Can you work these out from the model? Positions are in its coordinate system, mm. A direction names the side the tool comes from. Coordinates: 2 decimals unless noted, no trailing zeros. Loops run counter-clockwise (first coordinate to the right, second up) from the corner with the lowest first, then second, coordinate; pieces in that order, holes last.
```python
from build123d import *

# Parameters (mm, degrees)
BOX010_W          = 30
BOX010_H          = 9
BOX010_DEPTH      = 15
BOX011_W          = 31.5
BOX011_H          = 16
BOX011_DEPTH      = 12
CYLINDER_R        = 1.75
CYLINDER_DEPTH    = 10
CYLINDER001_R     = 1.75
CYLINDER001_DEPTH = 10
BOX009_W          = 44
BOX009_H          = 3
BOX009_DEPTH      = 17


with BuildPart() as cube010:
    # Box010 → Box010 (new body)
    with BuildSketch(Plane(origin=(43, -107, 23), x_dir=(1, 0, 0), z_dir=(0, 0, 1))):
        with Locations((15, 4.5)):
            Rectangle(BOX010_W, BOX010_H)
    extrude(amount=BOX010_DEPTH)


with BuildPart() as cube011:
    # Box011 → Box011 (new body)
    with BuildSketch(Plane(origin=(42, -95, 22), x_dir=(1, 0, 0), z_dir=(0, 0, 1))):
        with Locations((15.75, 8)):
            Rectangle(BOX011_W, BOX011_H)
    extrude(amount=BOX011_DEPTH)


with BuildPart() as cylinder:
    # Cylinder → Cylinder (new body)
    with BuildSketch(Plane(origin=(40, -91, 26.5), x_dir=(1, 0, 0), z_dir=(0, -1, 0))):
        Circle(CYLINDER_R)
    extrude(amount=CYLINDER_DEPTH)


with BuildPart() as fusion003:
    # Cylinder001 → Cylinder001 (new body)
    with BuildSketch(Plane(origin=(76.5, -91, 26.5), x_dir=(1, 0, 0), z_dir=(0, -1, 0))):
        Circle(CYLINDER001_R)
    extrude(amount=CYLINDER001_DEPTH)

    # Fusion003: union Cylinder
    add(cylinder.part)


with BuildPart() as fusion003_1:
    # Fusion003 placement: moved
    add(fusion003.part.moved(Location((-0.5, 0, 0))))


with BuildPart() as f_4p:
    # Box009 → Box009 (new body)
    with BuildSketch(Plane(origin=(36, -98, 19), x_dir=(1, 0, 0), z_dir=(0, 0, 1))):
        with Locations((22, 1.5)):
            Rectangle(BOX009_W, BOX009_H)
    extrude(amount=BOX009_DEPTH)

    # Fusion004: union Cube010, Cube011, Fusion003
    add(cube010.part)
    add(cube011.part)
    add(fusion003_1.part)


with BuildPart() as f_4p_1:
    # Fusion004 placement: moved
    add(f_4p.part.moved(Location((-5, 0, 0))))


solid = f_4p_1.part
```
Item 1: Suppose I cut it at C-C, the plane x = 34.5. Please give me the cut outline in (y, z), plus the area to 3 significant figures.
Results are:
outline: (-101, 24.75) - (-98, 24.75) - (-98, 19) - (-95, 19) - (-95, 24.75) - (-91, 24.75) - (-91, 28.25) - (-95, 28.25) - (-95, 36) - (-98, 36) - (-98, 28.25) - (-101, 28.25) - close
area: 75.5 mm2
Item 2: Suppose I cut it at B-B, the plane y = -100.5. Please give me the cut outline in (x, z), plus the area to 3 significant figures.
Results are:
outline: circle Ø3.5 at (34.5, 26.5); (38, 23) - (68, 23) - (68, 38) - (38, 38) - close; circle Ø3.5 at (71, 26.5)
area: 469 mm2
Item 3: I need wall thicknesses on line 1 along Z through (x, y) = (59.5, -99); line 2 along Z through (x, y) = (68, -88.5); line 3 along X through (y, z) = (-91, 24.5). Which ranges of each line are inside material? Lowest first, please.
Results are:
line 1: z = 23 to 38
line 2: z = 22 to 34
line 3: x = 37 to 68.5
Item 4: I'm going to push flat-ended pins straight in: P1, Ø4, axis at y = -86.5, z = 34, coming from the -X side; P2, Ø10, axis at y = -84.5, z = 24.5, coming from the +X side; P3, Ø1.8, axis at x = 34.5, z = 26.5, coming from the +Y side; P4, Ø2.5, axis at x = 49.5, y = -97, coming from the +Z side. Where does each tip first touch, or does it pass through?
Results are:
P1: stops at x = 37
P2: stops at x = 68.5
P3: stops at y = -91
P4: stops at z = 38
Item 5: Suppose I cut it at A-A, the plane z = 29.5. Please give me the cut outline in (x, y), plus the area to 3 significant figures.
Results are:
outline: (31, -98) - (38, -98) - (38, -107) - (68, -107) - (68, -98) - (75, -98) - (75, -95) - (68.5, -95) - (68.5, -79) - (37, -79) - (37, -95) - (31, -95) - close
area: 906 mm2
Item 6: We'd pull the mould along X, two halves only. Please class faces 5 (the face through (75, -97, 27)), 6 (the face through (34, -91, 27)), 7 (the face through (72.669, -99.479, 27.026)): +X half, -X half, draft (parallel to the pull), parting line (faces both ways), or undercut.
Results are:
face 5: +X half
face 6: draft
face 7: undercut
Item 7: On a 3-axis mill with a long thin cutter (end or side, diameter ignored), from which of +Z, -Z, +X, -X, +Y, -Y can I reach the whole of each face in a straight line? I mean faces 1 (the face through (33.21, -92.97, 27.68)), 2 (the face through (53, -96, 36)), 3 (the face through (71, -91, 27)), 4 (the face through (53, -102, 23)). Say none if no direction works.
Results are:
face 1: +Y
face 2: +Z, +X, -X, +Y
face 3: +Z, -Z, +X, +Y
face 4: -Z, +X, -X, -Y
Item 8: Suppose I cut it at D-D, the plane z = 26.5. Please give me the cut outline in (x, y), plus the area to 3 significant figures.
Results are:
outline: (31, -98) - (32.75, -98) - (32.75, -101) - (36.25, -101) - (36.25, -98) - (38, -98) - (38, -107) - (68, -107) - (68, -98) - (69.25, -98) - (69.25, -101) - (72.75, -101) - (72.75, -98) - (75, -98) - (75, -95) - (72.75, -95) - (72.75, -91) - (69.25, -91) - (69.25, -95) - (68.5, -95) - (68.5, -79) - (37, -79) - (37, -95) - (36.25, -95) - (36.25, -91) - (32.75, -91) - (32.75, -95) - (31, -95) - close
area: 955 mm2
